Design review of the part shown in the three views and the two pictorial views. Dimensions are in mm from the part's minimum x, y and z. A direction names the side the tool comes from. Give positions to 0.01 mm unless a question says otherwise; leave off trailing zeros. Loops run counter-clockwise (first coordinate to the right, second up) from the corner with the lowest first, then second, coordinate; pieces in that order, holes last. Notation, with made-up numbers: (22.5, -14) - (57.5, -14) arc R26 cw to (57.5, 8) - close; hole circle Ø11 at (-39, -39.75). An arc over 180 degrees is marked (long way). Answer as a JSON object with one key per item and string values.
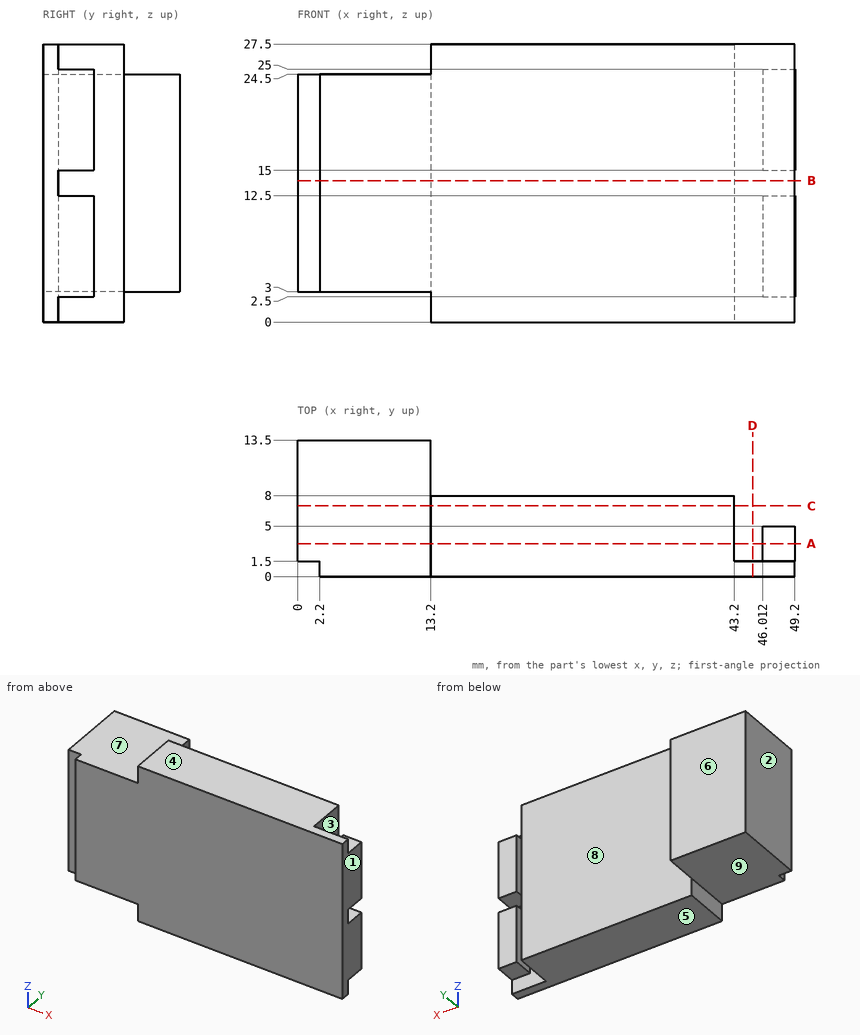
Q1. To check wall thickness, follow probe 1 along X at (y, z) = (2, 17.5); probe 2 along Z at (x, y) = (12, 7.25); probe 3 along Y at (x, z) = (37, 21.5). State the ranges of each line that lie inside material, in increasing order. Write a range as [from, to].
Results:
{"probe 1": "x = [0, 43.2], [46.01, 49.2]", "probe 2": "z = [3, 24.5]", "probe 3": "y = [0, 8]"}
Q2. The part is to be moulded in two halves that separate along X. For the marked faces 1, 2, 3 and 4, say which applies: +X half, -X half, draft (parallel to the pull), parting line (faces both ways), or undercut.
Results:
{"face 1": "+X half", "face 2": "-X half", "face 3": "undercut", "face 4": "draft"}
Q3. Clearance check with flat-ended pins moving along their axes: pin 1 Ø1.5 at (y, z) = (2.5, 26) entering from -X; pin 2 Ø2.5 at (x, z) = (47.5, 22) entering from +Y; pin 3 Ø0.8 at (y, z) = (0.5, 13) entering from -X. State where each tip first meets the part, or that it passes through.
Results:
{"pin 1": "stops at x = 13.2", "pin 2": "stops at y = 5", "pin 3": "stops at x = 2.2"}
Q4. Consider section A-A, the plane y = 3.25. State the section outline as (x, z) points, plus the area to 3 significant figures.
Results:
{"outline": "(0, 3) - (13.2, 3) - (13.2, 0) - (43.2, 0) - (43.2, 27.5) - (13.2, 27.5) - (13.2, 24.5) - (0, 24.5) - close; (46.01, 2.5) - (49.2, 2.5) - (49.2, 12.5) - (46.01, 12.5) - close; (46.01, 15) - (49.2, 15) - (49.2, 25) - (46.01, 25) - close", "area": "1,170 mm^2"}
Q5. Consider section C-C, the plane y = 7. State the section outline as (x, z) points, plus the area to 3 significant figures.
Results:
{"outline": "(0, 3) - (13.2, 3) - (13.2, 0) - (43.2, 0) - (43.2, 27.5) - (13.2, 27.5) - (13.2, 24.5) - (0, 24.5) - close", "area": "1,110 mm^2"}
Q6. For the marked faces 5, 6, 7, 8 and 9, list the 3-axis set-ups (+Z, -Z, +X, -X, +Y, -Y) from which the entire face can be reached by the end or side of a thin tool; tool diameter is ignored.
Results:
{"face 5": "-Z, +X, -X, +Y, -Y", "face 6": "+Z, -Z, +X, -X, +Y", "face 7": "+Z, -X, +Y, -Y", "face 8": "+Z, -Z, +X, +Y", "face 9": "-Z, -X, +Y, -Y"}
Q7. Consider section B-B, the plane z = 14. State the section outline as (x, y) points.
Results:
{"outline": "(0, 1.5) - (2.2, 1.5) - (2.2, 0) - (49.2, 0) - (49.2, 1.5) - (43.2, 1.5) - (43.2, 8) - (13.2, 8) - (13.2, 13.5) - (0, 13.5) - close"}
Q8. Consider section D-D, the plane x = 45. State the section outline as (y, z) points.
Results:
{"outline": "(0, 0) - (1.5, 0) - (1.5, 27.5) - (0, 27.5) - close"}
